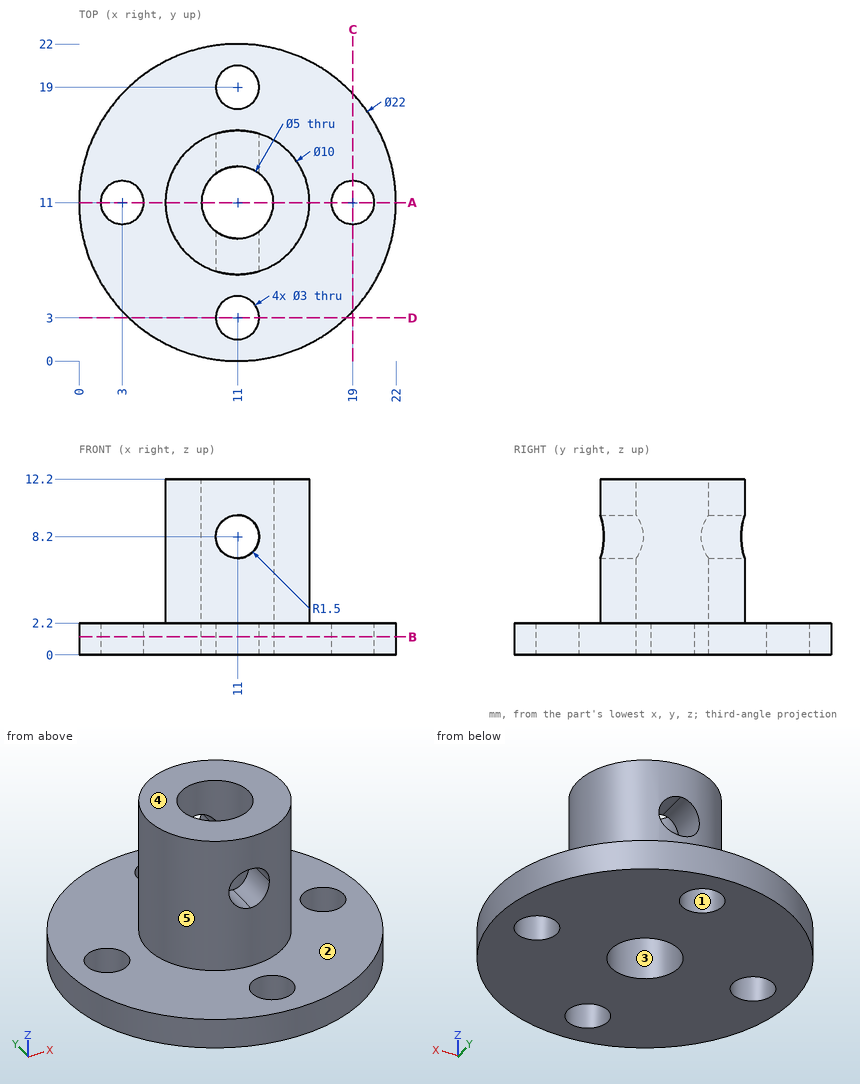
Geometry check sheet. Reference: drawing and pictorial views, mm from the part's lowest x, y, z. A direction names the side the tool comes from. Coordinates: 2 decimals unless noted, no trailing zeros. Order: outer loops, then holes, each group sorted by start corner. A loop starts at its lowest first (then second) coordinate and runs counter-clockwise, first axis right, second up. Notation, with made-up numbers: (14.25, 21.25) -> (63.25, 21.25) arc R19 cw to (63.25, 39.25) -> close; hole circle Ø9 at (-14.75, -9.75). An arc over 180 degrees is marked (long way). Put each result on its own line as item: value. Start each with the question number.
1) Material ranges on L1, parallel to Y at x = 11, z = 2.75; L2, parallel to Z at x = 6, y = 4; L3, parallel to Z at x = 10.5, y = 13.5, recorded low to high.
2) Go/stop test with flat-tipped pins: pin 1 (5 mm diameter, centred on x = 11, y = 19, fed in from +Z); pin 2 (3 mm diameter, centred on y = 4, z = 3, fed in from +X); pin 3 (1.5 mm diameter, centred on y = 8.5, z = 2, fed in from -X). Record where each tip stops, or that it passes through.
3) Release check for a two-part mould opening along X. For the marked faces 3, 4 and 5 record: pulls with the +X half, pulls with the -X half, needs draft (parallel to the pull), parting line crosses it, or undercut.
4) Cross-section at A-A (y = 11). Enter the section's corners in (x, z).
5) Cross-section at C-C (x = 19). Enter the section's corners in (y, z), plus the area to 3 significant figures.
6) Cross-section at B-B (z = 1.25). Enter the section's corners in (x, y), plus the area to 3 significant figures.
7) Tool access check on the marked faces 1 and 2. Record the directions out of +Z, -Z, +X, -X, +Y, -Y that give a thin tool (end or side, any length) a straight path to the whole face; none if there is none.
Geometry check:
1. L1: y = 6 to 8.5, 13.5 to 16
1. L2: z = 0 to 2.2
1. L3: z = 0 to 6.79, 9.61 to 12.2
2. pin 1: stops at z = 2.2
2. pin 2: stops at x = 20.39
2. pin 3: stops at x = 0.14
3. face 3: undercut
3. face 4: needs draft
3. face 5: parting line crosses it
4. outline: (0, 0) -> (1.5, 0) -> (1.5, 2.2) -> (0, 2.2) -> close; (4.5, 0) -> (8.5, 0) -> (8.5, 12.2) -> (6, 12.2) -> (6, 2.2) -> (4.5, 2.2) -> close; (13.5, 0) -> (17.5, 0) -> (17.5, 2.2) -> (16, 2.2) -> (16, 12.2) -> (13.5, 12.2) -> close; (20.5, 0) -> (22, 0) -> (22, 2.2) -> (20.5, 2.2) -> close
5. outline: (3.45, 0) -> (9.5, 0) -> (9.5, 2.2) -> (3.45, 2.2) -> close; (12.5, 0) -> (18.55, 0) -> (18.55, 2.2) -> (12.5, 2.2) -> close
5. area: 26.6 mm^2
6. outline: circle Ø22 at (11, 11); hole circle Ø3 at (3, 11); hole circle Ø5 at (11, 11); hole circle Ø3 at (11, 3); hole circle Ø3 at (11, 19); hole circle Ø3 at (19, 11)
6. area: 332 mm^2
7. face 1: +Z, -Z
7. face 2: +Z
